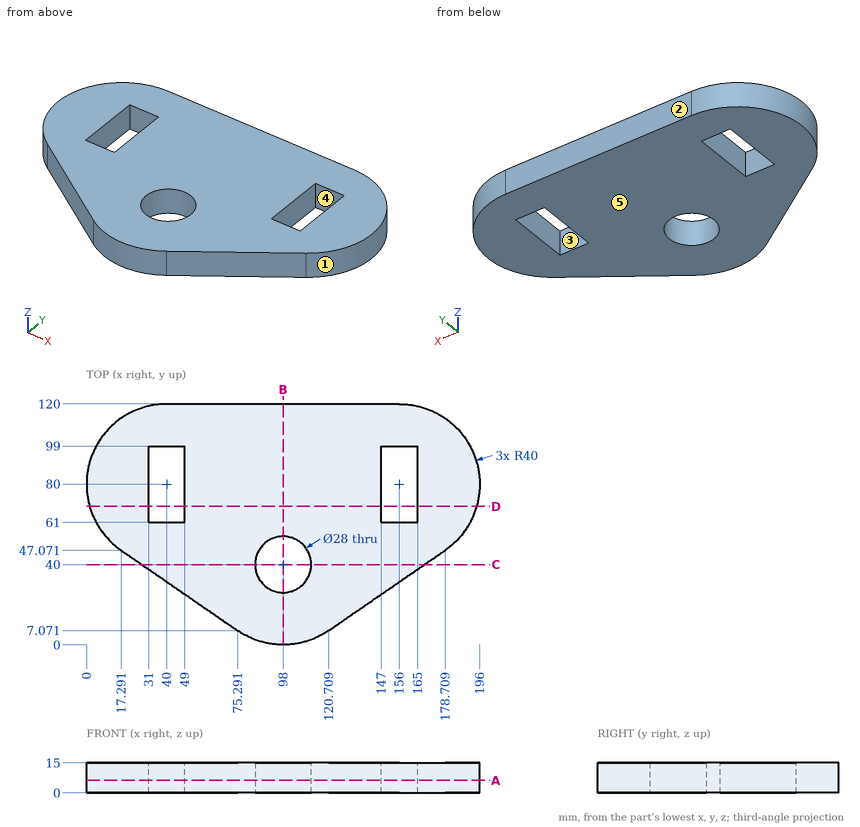
Design review of the part shown in the three views and the two pictorial views. Dimensions are in mm from the part's minimum x, y and z. A direction names the side the tool comes from. Round coordinates to 2 decimals unless told otherwise and drop trailing zeros. Loops run counter-clockwise (first coordinate to the right, second up) from the corner with the lowest first, then second, coordinate; pieces in that order, holes last. Notation, with made-up numbers: (33.25, 46) -> (81.25, 46) arc R28 ccw to (81.25, 76) -> close; hole circle Ø9 at (88.25, 68.25). An arc over 180 degrees is marked (long way). Use one line per item in the form item = value. Start each with the question number.
Q1. We need section C-C on y = 40. Give the boundary of the cut face in (x, z) (1 decimal), then the cut area to 3 significant figures.
Q2. Draft analysis for pull direction X (two halves, no side actions). For the marked faces 1, 2 and 3, state which applies: +X half, -X half, draft (parallel to the pull), parting line (faces both ways), or undercut.
Q3. We need section A-A on z = 6.25. Give the boundary of the cut face in (x, y).
Q4. We need section D-D on y = 69. Give the boundary of the cut face in (x, z).
Q5. We need section B-B on x = 98. Give the boundary of the cut face in (y, z), then the cut area to 3 significant figures.
Q6. Wall thickness on line 1 along Y through (x, z) = (98, 4.5); line 2 along X through (y, z) = (69, 7.25); line 3 along X through (y, z) = (73, 1): over which ranges is each line inside the solid? List them lowest first. Write a range as [from, to].
Q7. For pin 1 Ø1.5 at (x, z) = (38.5, 7.5) entering from +Y; pin 2 Ø6 at (y, z) = (27, 8) entering from -X (1 decimal); pin 3 Ø1 at (x, z) = (170.5, 7) entering from -Y (1 decimal), all flat-tipped, find the tip position at first contact; note any pin that passes through.
Q8. Machinability: for the marked faces 4 and 5, which of the approach directions +Z, -Z, +X, -X, +Y, -Y give a long, thin tool a straight path to every point of the face, cutting with its end or side? Answer none if there is none.
Calculated:
q1.outline = (27.5, 0) -> (84, 0) -> (84, 15) -> (27.5, 15) -> close; (112, 0) -> (168.5, 0) -> (168.5, 15) -> (112, 15) -> close
q1.area = 1,690 mm²
q2.face_1 = +X half
q2.face_2 = draft
q2.face_3 = undercut
q3.outline = (17.29, 47.07) -> (75.29, 7.07) arc R40 ccw to (120.71, 7.07) -> (178.71, 47.07) arc R40 ccw to (156, 120) -> (40, 120) arc R40 ccw to start; hole (31, 61) -> (49, 61) -> (49, 99) -> (31, 99) -> close; hole circle Ø28 at (98, 40); hole (147, 61) -> (165, 61) -> (165, 99) -> (147, 99) -> close
q4.outline = (1.54, 0) -> (31, 0) -> (31, 15) -> (1.54, 15) -> close; (49, 0) -> (147, 0) -> (147, 15) -> (49, 15) -> close; (165, 0) -> (194.46, 0) -> (194.46, 15) -> (165, 15) -> close
q5.outline = (0, 0) -> (26, 0) -> (26, 15) -> (0, 15) -> close; (54, 0) -> (120, 0) -> (120, 15) -> (54, 15) -> close
q5.area = 1,380 mm²
q6.line_1 = [0, 26], [54, 120]
q6.line_2 = [1.54, 31], [49, 147], [165, 194.46]
q6.line_3 = [0.62, 31], [49, 147], [165, 195.38]
q7.pin_1 = 119.99
q7.pin_2 = 42
q7.pin_3 = 41.1
q8.face_4 = +Z, -Z
q8.face_5 = -Z, +X, -X, +Y, -Y
